Read the model definition and answer for the solid it produces. Units are mm, in the model's axes. A direction names the side the tool comes from. Coordinates: 2 decimals unless noted, no trailing zeros. Order: outer loops, then holes, each group sorted by start corner. A loop starts at its lowest first (then second) coordinate and runs counter-clockwise, first axis right, second up.
from build123d import *

# Parameters (mm, degrees)
EXTRUDE_1_DEPTH     = 52
SKETCH_3_W          = 28
SKETCH_3_H          = 52
EXTRUDE_2_DEPTH     = 3.5
CUT_EXTRUDE_1_REACH = 66.84
SKETCH_4_R          = 1.6
SKETCH_6_R          = 7
CUT_EXTRUDE_2_DEPTH = 65.840188155
SKETCH_7_R          = 4
CUT_EXTRUDE_3_DEPTH = 1.2
CUT_EXTRUDE_4_REACH = 66.712


with BuildPart() as part:
    # 草图2 → 凸台-拉伸1 (new body)
    with BuildSketch(Plane(origin=(0, 0, 0), x_dir=(1, 0, 0), z_dir=(0, 1, 0))):
        Polygon((0, 0), (38, 0), (35, 4), (3, 4), align=None)
    extrude(amount=EXTRUDE_1_DEPTH)

    # 草图3 → 凸台-拉伸2 (add)
    with BuildSketch(Plane(origin=(0, 0, -4), x_dir=(-1, 0, 0), z_dir=(0, 0, -1))):
        with Locations((-19, 26)):
            Rectangle(SKETCH_3_W, SKETCH_3_H)
    extrude(amount=EXTRUDE_2_DEPTH)

    # 草图4 → 切除-拉伸1 (cut, up to next)
    with BuildSketch(Plane.XY, mode=Mode.PRIVATE) as cut_extrude_1_sk1:
        with Locations((8, 3.25)):
            Circle(SKETCH_4_R)
    cut_extrude_1_tool1 = extrude(cut_extrude_1_sk1.sketch, amount=-CUT_EXTRUDE_1_REACH, mode=Mode.PRIVATE) & part.part
    # 草图4 → 切除-拉伸1 (cut, up to next)
    with BuildSketch(Plane.XY, mode=Mode.PRIVATE) as cut_extrude_1_sk2:
        with Locations((30, 3.25)):
            Circle(SKETCH_4_R)
    cut_extrude_1_tool2 = extrude(cut_extrude_1_sk2.sketch, amount=-CUT_EXTRUDE_1_REACH, mode=Mode.PRIVATE) & part.part
    # 草图4 → 切除-拉伸1 (cut, up to next)
    with BuildSketch(Plane.XY, mode=Mode.PRIVATE) as cut_extrude_1_sk3:
        with Locations((8, 48.75)):
            Circle(SKETCH_4_R)
    cut_extrude_1_tool3 = extrude(cut_extrude_1_sk3.sketch, amount=-CUT_EXTRUDE_1_REACH, mode=Mode.PRIVATE) & part.part
    # 草图4 → 切除-拉伸1 (cut, up to next)
    with BuildSketch(Plane.XY, mode=Mode.PRIVATE) as cut_extrude_1_sk4:
        with Locations((27, 48.75)):
            Circle(SKETCH_4_R)
    cut_extrude_1_tool4 = extrude(cut_extrude_1_sk4.sketch, amount=-CUT_EXTRUDE_1_REACH, mode=Mode.PRIVATE) & part.part
    add(cut_extrude_1_tool1.solids().sort_by_distance((8, 3.25, 0))[0], mode=Mode.SUBTRACT)
    add(cut_extrude_1_tool2.solids().sort_by_distance((30, 3.25, 0))[0], mode=Mode.SUBTRACT)
    add(cut_extrude_1_tool3.solids().sort_by_distance((8, 48.75, 0))[0], mode=Mode.SUBTRACT)
    add(cut_extrude_1_tool4.solids().sort_by_distance((27, 48.75, 0))[0], mode=Mode.SUBTRACT)

    # 草图6 → 切除-拉伸2 (cut, through all)
    with BuildSketch(Plane.XY):
        with Locations((19, 0.05)):
            Circle(SKETCH_6_R)
    extrude(amount=-CUT_EXTRUDE_2_DEPTH, mode=Mode.SUBTRACT)

    # 草图7 → 切除-拉伸3 (cut)
    with BuildSketch(Plane.XY):
        with Locations((8, 48.75)):
            Circle(SKETCH_7_R)
        with Locations((27, 48.75)):
            Circle(SKETCH_7_R)
        with Locations((8, 3.25)):
            Circle(SKETCH_7_R)
        with Locations((30, 3.25)):
            Circle(SKETCH_7_R)
    extrude(amount=-CUT_EXTRUDE_3_DEPTH, mode=Mode.SUBTRACT)

    # 草图8 → 切除-拉伸4 (cut, up to next)
    with BuildSketch(Plane.XY.offset(-1.2), mode=Mode.PRIVATE) as cut_extrude_4_sk1:
        with BuildLine():
            Line((3.8, 48.75), (3.8, 52))
            ThreePointArc((3.8, 52), (8, 56.2), (12.2, 52))
            Line((12.2, 52), (12.2, 48.75))
            ThreePointArc((12.2, 48.75), (8, 44.55), (3.8, 48.75))
        make_face()
    cut_extrude_4_tool1 = extrude(cut_extrude_4_sk1.sketch, amount=CUT_EXTRUDE_4_REACH, mode=Mode.PRIVATE) & part.part
    # 草图8 → 切除-拉伸4 (cut, up to next)
    with BuildSketch(Plane.XY.offset(-1.2), mode=Mode.PRIVATE) as cut_extrude_4_sk2:
        with BuildLine():
            Line((22.8, 48.75), (22.8, 52))
            ThreePointArc((22.8, 52), (27, 56.2), (31.2, 52))
            Line((31.2, 52), (31.2, 48.75))
            ThreePointArc((31.2, 48.75), (27, 44.55), (22.8, 48.75))
        make_face()
    cut_extrude_4_tool2 = extrude(cut_extrude_4_sk2.sketch, amount=CUT_EXTRUDE_4_REACH, mode=Mode.PRIVATE) & part.part
    # 草图8 → 切除-拉伸4 (cut, up to next)
    with BuildSketch(Plane.XY.offset(-1.2), mode=Mode.PRIVATE) as cut_extrude_4_sk3:
        with BuildLine():
            Line((12.2, 3.25), (12.2, 0))
            ThreePointArc((12.2, 0), (8, -4.2), (3.8, 0))
            Line((3.8, 0), (3.8, 3.25))
            ThreePointArc((3.8, 3.25), (8, 7.45), (12.2, 3.25))
        make_face()
    cut_extrude_4_tool3 = extrude(cut_extrude_4_sk3.sketch, amount=CUT_EXTRUDE_4_REACH, mode=Mode.PRIVATE) & part.part
    # 草图8 → 切除-拉伸4 (cut, up to next)
    with BuildSketch(Plane.XY.offset(-1.2), mode=Mode.PRIVATE) as cut_extrude_4_sk4:
        with BuildLine():
            Line((34.2, 3.25), (34.2, 0))
            ThreePointArc((34.2, 0), (30, -4.2), (25.8, 0))
            Line((25.8, 0), (25.8, 3.25))
            ThreePointArc((25.8, 3.25), (30, 7.45), (34.2, 3.25))
        make_face()
    cut_extrude_4_tool4 = extrude(cut_extrude_4_sk4.sketch, amount=CUT_EXTRUDE_4_REACH, mode=Mode.PRIVATE) & part.part
    add(cut_extrude_4_tool1.solids().sort_by_distance((8, 50.375, -1.2))[0], mode=Mode.SUBTRACT)
    add(cut_extrude_4_tool2.solids().sort_by_distance((27, 50.375, -1.2))[0], mode=Mode.SUBTRACT)
    add(cut_extrude_4_tool3.solids().sort_by_distance((8, 1.625, -1.2))[0], mode=Mode.SUBTRACT)
    add(cut_extrude_4_tool4.solids().sort_by_distance((30, 1.625, -1.2))[0], mode=Mode.SUBTRACT)


solid = part.part
Q1. The part is cut by section A-A, the plane x = 8. Determine the outline of the cut face in (y, z).
Q2. The part is cut by section D-D, the plane x = 19. Determine the outline of the cut face in (y, z).
Q3. The part is cut by section C-C, the plane y = 24. Determine the outline of the cut face in (x, z), then the cut area to 3 significant figures.
Q4. Straight lines are drawn through the part: L1, parallel to Y at x = 8, z = -3; L2, parallel to Y at x = 30, z = -5.5; L3, parallel to X at y = 4.5, z = -7. For each, find the intervals that lie inside material, in ascending order.
Q5. Which of the six approach directions +Z, -Z, +X, -X, +Y, -Y give full straight-line access (tool end or side, diameter ignored) to faces 1 (the flat face through (9, 5, -1.2)), 2 (the flat face through (12.2, 50, -1)), 3 (the flat face through (4, 26, -4))?
Q6. Each of these flat-tipped pins is pushed along its axis until it touches: P1, Ø1, axis at y = 39, z = -5, coming from the -X side; P2, Ø1.8, axis at y = 38.5, z = -6.5, coming from the +X side; P3, Ø3, axis at y = 9, z = -4.5, coming from the +X side; P4, Ø2.5, axis at x = 8, y = 3.25, coming from the +Z side. Where does it stop, or does it pass through?
Q7. The part is cut by section B-B, the plane z = -2. Determine the outline of the cut face in (x, y).
Computed values:
1. outline: (0, -7.5) - (1.65, -7.5) - (1.65, -1.2) - (0, -1.2) - close; (4.85, -7.5) - (47.15, -7.5) - (47.15, -1.2) - (44.55, -1.2) - (44.55, 0) - (7.45, 0) - (7.45, -1.2) - (4.85, -1.2) - close; (50.35, -7.5) - (52, -7.5) - (52, -1.2) - (50.35, -1.2) - close
2. outline: (7.05, -7.5) - (52, -7.5) - (52, 0) - (7.05, 0) - close
3. outline: (0, 0) - (3, -4) - (5, -4) - (5, -7.5) - (33, -7.5) - (33, -4) - (35, -4) - (38, 0) - close
3. area: 238 mm2
4. L1: y = 0 to 1.65, 4.85 to 47.15, 50.35 to 52
4. L2: y = 0 to 1.65, 4.85 to 52
4. L3: x = 5 to 7, 9 to 13.6, 24.4 to 29, 31 to 33
5. face 1: +Z, -Y
5. face 2: +Z, +Y
5. face 3: -Z, -X, +Y, -Y
6. P1: stops at x = 5
6. P2: stops at x = 33
6. P3: stops at x = 35.75
6. P4: passes through
7. outline: (1.5, 0) - (12, 0) arc R7 cw (long way) to (26, 0) - (36.5, 0) - (36.5, 52) - (1.5, 52) - close; hole circle Ø3.2 at (8, 3.25); hole circle Ø3.2 at (8, 48.75); hole circle Ø3.2 at (27, 48.75); hole circle Ø3.2 at (30, 3.25)
